For this review, take the finished solid that the model builds, in its own axes (mm). Give positions to 0.01 mm unless a question says otherwise; leave off trailing zeros. Order: outer loops, then holes, each group sorted by start corner. A loop starts at its lowest first (then second) coordinate and runs counter-clockwise, first axis right, second up.
from build123d import *

# Parameters (mm, degrees)
SKETCH1_R           = 2.6
BOSS_EXTRUDE1_DEPTH = 3.175
SKETCH2_R           = 2.54
CUT_EXTRUDE1_DEPTH  = 10


with BuildPart() as part:
    # Sketch1 → Boss-Extrude1 (new body)
    with BuildSketch(Plane(origin=(0, 0, 0), x_dir=(1, 0, 0), z_dir=(0, 1, 0))):
        with BuildLine():
            ThreePointArc((-17.206636662, 27.922333563), (-28.354981926, 28.354981926), (-27.922333563, 17.206636662))
            ThreePointArc((-27.922333563, 17.206636662), (-20, 0), (-27.922333563, -17.206636662))
            ThreePointArc((-27.922333563, -17.206636662), (-28.354981926, -28.354981926), (-17.206636662, -27.922333563))
            ThreePointArc((-17.206636662, -27.922333563), (0, -20), (17.206636662, -27.922333563))
            ThreePointArc((17.206636662, -27.922333563), (28.354981926, -28.354981926), (27.922333563, -17.206636662))
            ThreePointArc((27.922333563, -17.206636662), (20, 0), (27.922333563, 17.206636662))
            ThreePointArc((27.922333563, 17.206636662), (28.354981926, 28.354981926), (17.206636662, 27.922333563))
            ThreePointArc((17.206636662, 27.922333563), (0, 20), (-17.206636662, 27.922333563))
        make_face()
        with Locations(Location((22.980970389, 22.980970389, 0), (0, 0, 270))):
            Circle(SKETCH1_R, mode=Mode.SUBTRACT)
        with Locations(Location((22.980970389, -22.980970389, 0), (0, 0, 270))):
            Circle(SKETCH1_R, mode=Mode.SUBTRACT)
        with Locations(Location((-22.980970389, -22.980970389, 0), (0, 0, 270))):
            Circle(SKETCH1_R, mode=Mode.SUBTRACT)
        with Locations(Location((-22.980970389, 22.980970389, 0), (0, 0, 270))):
            Circle(SKETCH1_R, mode=Mode.SUBTRACT)
        with BuildLine():
            Line((2.353261567, 13.359444444), (-2.353261567, 13.359444444))
            Line((-2.353261567, 13.359444444), (-2.353261567, 11.113016606))
            ThreePointArc((-2.353261567, 11.113016606), (0, -11.359444444), (2.353261567, 11.113016606))
            Line((2.353261567, 11.113016606), (2.353261567, 13.359444444))
        make_face(mode=Mode.SUBTRACT)
    extrude(amount=BOSS_EXTRUDE1_DEPTH)

    # Sketch2 → Cut-Extrude1 (cut)
    with BuildSketch(Plane(origin=(0, 3.175, 0), x_dir=(1, 0, 0), z_dir=(0, 1, 0))):
        with Locations(Location((-5.08, -15.679722222, 0), (0, 0, 270))):
            Circle(SKETCH2_R)
        with Locations(Location((5.08, -15.679722222, 0), (0, 0, 270))):
            Circle(SKETCH2_R)
    extrude(amount=-CUT_EXTRUDE1_DEPTH, mode=Mode.SUBTRACT)


solid = part.part
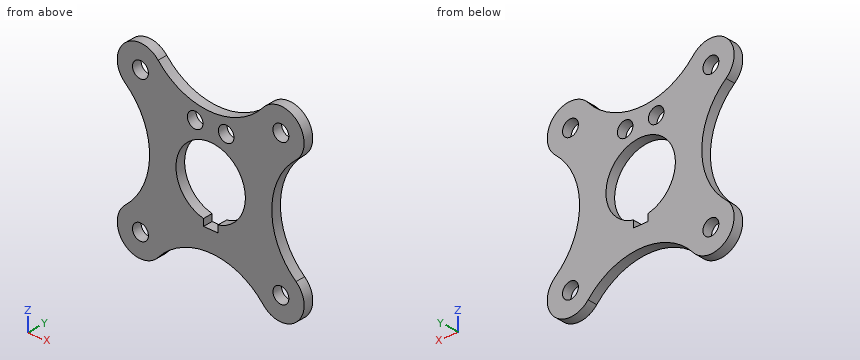
1) We need section D-D on y = 2. Give the boundary of the cut face in (x, z), then the cut area to 3 significant figures.
Answer sheet:
outline: (-27.92, -17.21) arc R7.6 ccw (long way) to (-17.21, -27.92) arc R22.65 cw to (17.21, -27.92) arc R7.6 ccw (long way) to (27.92, -17.21) arc R22.65 cw to (27.92, 17.21) arc R7.6 ccw (long way) to (17.21, 27.92) arc R22.65 cw to (-17.21, 27.92) arc R7.6 ccw (long way) to (-27.92, 17.21) arc R22.65 cw to start; hole circle Ø5.2 at (-22.98, -22.98); hole circle Ø5.2 at (-22.98, 22.98); hole circle Ø5.08 at (-5.08, 15.68); hole (-2.35, -13.36) - (2.35, -13.36) - (2.35, -11.11) arc R11.36 ccw (long way) to (-2.35, -11.11) - close; hole circle Ø5.08 at (5.08, 15.68); hole circle Ø5.2 at (22.98, -22.98); hole circle Ø5.2 at (22.98, 22.98)
area: 1,990 mm2
2) We need section A-A on x = 0. Give the boundary of the cut face in (y, z) (3 decimals), then the cut area to 3 significant figures.
Answer sheet:
outline: (0, -20) - (3.175, -20) - (3.175, -13.359) - (0, -13.359) - close; (0, 11.359) - (3.175, 11.359) - (3.175, 20) - (0, 20) - close
area: 48.5 mm2
3) We need section B-B on z = 15. Give the boundary of the cut face in (x, y) (3 decimals).
Answer sheet:
outline: (-25.68, 0) - (-7.527, 0) - (-7.527, 3.175) - (-25.68, 3.175) - close; (-2.633, 0) - (2.633, 0) - (2.633, 3.175) - (-2.633, 3.175) - close; (7.527, 0) - (25.68, 0) - (25.68, 3.175) - (7.527, 3.175) - close
4) To check wall thickness, follow line 1 (Z direction, x = 22.5, y = 2.9); line 2 (Z direction, x = 3.5, y = 0.85); line 3 (X direction, y = 1.8, z = 25). State the ranges of each line that lie inside material, in increasing order.
Answer sheet:
line 1: z = -30.57 to -25.54, -20.43 to -10.34, 10.34 to 20.43, 25.54 to 30.57
line 2: z = -20.27 to -10.81, 10.81 to 13.69, 17.67 to 20.27
line 3: x = -30.31 to -24.62, -21.34 to -14.19, 14.19 to 21.34, 24.62 to 30.31
5) We need section C-C on z = 0. Give the boundary of the cut face in (x, y) (3 decimals), then the cut area to 3 significant figures.
Answer sheet:
outline: (-20, 0) - (-11.359, 0) - (-11.359, 3.175) - (-20, 3.175) - close; (11.359, 0) - (20, 0) - (20, 3.175) - (11.359, 3.175) - close
area: 54.9 mm2
6) Clearance check with flat-ended pins moving along their axes: pin 1 (1 mm diameter, centred on y = 1.5, z = 6.5, fed in from +X); pin 2 (0.7 mm diameter, centred on y = 1.5, z = -12, fed in from -X); pin 3 (12 mm diameter, centred on x = -6.5, z = -3, fed in from +Y) (3 decimals). State where each tip first meets the part, or that it passes through.
Answer sheet:
pin 1: stops at x = 21.11
pin 2: stops at x = -23.66
pin 3: stops at y = 3.175
